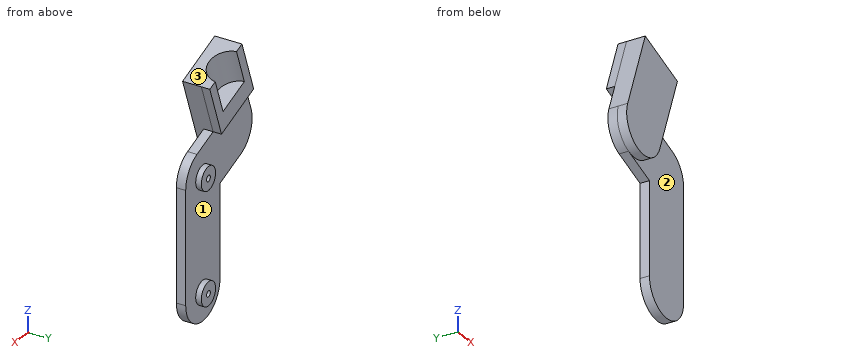
from build123d import *

# Parameters (mm, degrees)
EXTRUDE_1_DEPTH        = 5
SKETCH_2_R             = 6.25
EXTRUDE_2_DEPTH        = 3
HOLE_WIZARD_M4_1_D     = 3.3
HOLE_WIZARD_M4_1_DEPTH = 5
HOLE_WIZARD_M4_1_TIP   = 0.991420021
EXTRUDE_3_DEPTH        = 5
EXTRUDE_4_DEPTH        = 5
EXTRUDE_4_DEPTH_BACK   = 5
EXTRUDE_5_DEPTH        = 4.5
SKETCH_12_R            = 10
CUT_EXTRUDE_1_DEPTH    = 20


with BuildPart() as part:
    # Sketch 1 → Extrude 1 (new body)
    with BuildSketch(Plane(origin=(0, 0, 0), x_dir=(1, 0, 0), z_dir=(0, 1, 0))):
        with BuildLine():
            Line((-15, 0), (-15, 60))
            ThreePointArc((-15, 60), (0, 75), (15, 60))
            Line((15, 60), (15, 0))
            ThreePointArc((15, 0), (0, -15), (-15, 0))
        make_face()
    extrude(amount=EXTRUDE_1_DEPTH)

    # Sketch 2 → Extrude 2 (add)
    with BuildSketch(Plane(origin=(0, 5, 0), x_dir=(1, 0, 0), z_dir=(0, 1, 0))):
        with Locations((0, 60)):
            Circle(SKETCH_2_R)
        Circle(SKETCH_2_R)
    extrude(amount=EXTRUDE_2_DEPTH)

    # Hole Wizard M4 _ _ _ _1
    with Locations(Plane(origin=(0, 8, 0), x_dir=(1, 0, 0), z_dir=(0, 1, 0))):
        with Locations((0, 0), (0, 60)):
            Hole(HOLE_WIZARD_M4_1_D / 2, depth=HOLE_WIZARD_M4_1_DEPTH)
            with Locations((0, 0, -(HOLE_WIZARD_M4_1_DEPTH + HOLE_WIZARD_M4_1_TIP / 2))):  # 118° drill point
                Cone(0, HOLE_WIZARD_M4_1_D / 2, HOLE_WIZARD_M4_1_TIP, mode=Mode.SUBTRACT)

    # Sketch 9 → Extrude 3 (add)
    with BuildSketch(Plane.XZ):
        with BuildLine():
            Line((-5.13030215, -14.095389312), (-33.321080773, -3.834785012))
            ThreePointArc((-33.321080773, -3.834785012), (-42.286167935, 15.39090645), (-23.060476474, 24.355993612))
            Line((-23.060476474, 24.355993612), (5.13030215, 14.095389312))
            ThreePointArc((5.13030215, 14.095389312), (14.095389312, -5.13030215), (-5.13030215, -14.095389312))
        make_face()
    extrude(amount=-EXTRUDE_3_DEPTH)

    # Sketch 10 → Extrude 4 (add, two sides)
    with BuildSketch(Plane.XZ) as extrude_4_sk:
        with BuildLine():
            Line((-42.286167935, 15.39090645), (-26.895261486, 57.677074385))
            Line((-26.895261486, 57.677074385), (1.295517138, 47.416470085))
            Line((1.295517138, 47.416470085), (-14.095389312, 5.13030215))
            ThreePointArc((-14.095389312, 5.13030215), (-33.321080773, -3.834785012), (-42.286167935, 15.39090645))
        make_face()
    extrude(amount=EXTRUDE_4_DEPTH)
    extrude(extrude_4_sk.sketch, amount=-EXTRUDE_4_DEPTH_BACK)

    # Sketch 11 → Extrude 5 (add)
    with BuildSketch(Plane(origin=(0, 5, 0), x_dir=(1, 0, 0), z_dir=(0, 1, 0))):
        Polygon((-26.895261486, -57.677074385), (-37.155865785, -29.486295761), (-8.965087162, -19.225691462), (1.295517138, -47.416470085), align=None)
    extrude(amount=EXTRUDE_5_DEPTH)

    # Sketch 12 → Cut-Extrude 1 (cut)
    with BuildSketch(Plane(origin=(15.39090645, 0, 42.286167935), x_dir=(0.939692621, 0, -0.342020143), z_dir=(0.342020143, 0, 0.939692621))):
        with Locations((-30, 10.5)):
            Circle(SKETCH_12_R)
    extrude(amount=-CUT_EXTRUDE_1_DEPTH, mode=Mode.SUBTRACT)


solid = part.part
Can you work these out from the model? Positions are in its coordinate system, mm. Face numbers are marked on the shaded views. Give positions to 0.01 mm unless a question says otherwise; leave off trailing zeros. Order: outer loops, then holes, each group sorted by start corner. A loop starts at its lowest first (then second) coordinate and runs counter-clockwise, first axis right, second up. Notation, with made-up numbers: M 39.5,53 L 93.5,53 A12 ccw 93.5,57 Z; hole C 15.5,18.5 d1. An arc over 180 degrees is marked long. Use a Markdown table: item, result. Add a question column.
Item 1: Suppose I cut it at B-B (z = -15). List the corners of the cut face in (x, y) for me, then the cut area to 3 significant figures.
Item 2: Will these pins go through, and if not, where does the flat tip stop? pin 1 (8 mm diameter, centred on x = -13.5, z = 14, fed in from +Y); pin 2 (14 mm diameter, centred on x = 1.5, z = 3, fed in from +Y); pin 3 (14.5 mm diameter, centred on x = -9.5, z = -35.5, fed in from -Y).
Item 3: Suppose I cut it at A-A (y = -3). List the corners of the cut face in (x, z) for me, then the cut area to 3 significant figures.
Item 4: We'd pull the mould along Z, two halves only. Please class the marked faces 1, 2 and 3: +Z half, -Z half, draft (parallel to the pull), parting line (faces both ways), or undercut.
Item 5: If I drill on L1, parallel to X at y = 6.7, z = -60; L2, parallel to X at y = 4.7, z = -60; L3, parallel to Y at x = -10.5, z = 47.5, over which ranges is the centre line in solid material (lowest first)? Write a range as [from, to].
Answer sheet:
| question | item | result |
|---|---|---|
| 1 | outline | M -15,0 L 15,0 L 15,5 L -15,5 Z |
| 1 | area | 150 mm² |
| 2 | pin 1 | stops at y = 5 |
| 2 | pin 2 | stops at y = 8 |
| 2 | pin 3 | stops at y = 0 |
| 3 | outline | M -42.29,15.39 A15 ccw -14.1,5.13 L 1.3,47.42 L -26.9,57.68 Z |
| 3 | area | 1,700 mm² |
| 4 | face 1 | undercut |
| 4 | face 2 | draft |
| 4 | face 3 | +Z half |
| 5 | L1 | x = [-6.25, -1.65], [1.65, 6.25] |
| 5 | L2 | x = [-15, -1.65], [1.65, 15] |
| 5 | L3 | y = [-5, 1.29] |
